Geometry check sheet. Reference: the model listing, model coordinates, mm. A direction names the side the tool comes from. Give positions to 0.01 mm unless a question says otherwise; leave off trailing zeros. Write each loop counter-clockwise with the first axis right and the second up, starting at its lowest first coordinate (ties: lowest second). Pieces come first, ordered by that corner, then holes. Notation, with made-up numbers: (17, -3.5) - (41, -3.5) arc R10 ccw to (41, 14.5) - close; hole circle Ø1 at (30, 48.25). An arc over 180 degrees is marked (long way). One line per question, with ' | ' between items. Start each with the question number.
Q1. Set-up check for faces 1 (the face through (161.076, -36.429, 35.769)), 2 (the face through (66.538, 0.826, -34.608)), 3 (the face through (-129.48, -51.5, 134.64)): record each of +Z, -Z, +X, -X, +Y, -Y from which the full face is reachable in a straight line by a thin tool's end or side.
Q2. Section check B-B on x = -182. Record the boundary of the cut face in (y, z), and give its area (3 significant figures).
Q3. Release check for a two-part mould opening along X. For faces 4 (the face through (-69.12, -51.5, 162.17)), 5 (the face through (-25.532, 11.036, -81.075)), 6 (the face through (-134.64, -51.5, -129.48)), 7 (the face through (118, -56.569, 103)) record: +X half, -X half, draft (parallel to the pull), parting line (faces both ways), or undercut.
Q4. Section check A-A on z = 182. Record the boundary of the cut face in (x, y), and give its area (3 significant figures).
Q5. Section check C-C on y = -32. Record the boundary of the cut face in (x, z), and give its area (3 significant figures).
Q6. Thickness scan on L1, parallel to Y at x = 137.5, z = -113.5; L2, parallel to Y at x = 91, z = 84; L3, parallel to Z at x = 98, y = -16.5. Record the ranges inside material, lowest first. Write a range as [from, to].
Q7. Section check D-D on z = 0. Count the separate pieces of the cut face and the enclosed holes in it, and give its area (3 significant figures).
Q8. Gauge pin test, flat ends, axial feed: P1, Ø8, axis at x = 130, y = -20, coming from the +Z side; P2, Ø10, axis at x = 76.5, z = 120, coming from the +Y side; P3, Ø12, axis at x = 14.5, y = -26, coming from the -Z side. Record the tip position at first contact, or that the pin passes through.
```python
from build123d import *

# Parameters (mm, degrees)
SKETCH3_R          = 6
CUT_EXTRUDE1_DEPTH = 291.215437219
CIRPATTERN1_COUNT  = 16
SKETCH4_R          = 50
CUT_EXTRUDE2_DEPTH = 293.617497768


with BuildPart() as part:
    # Sketch2 → Revolve1 (revolve)
    with BuildSketch(Plane.XY, mode=Mode.PRIVATE) as revolve1_sk:
        with BuildLine():
            Line((155, -56.568542495), (200, -56.568542495))
            Line((200, -56.568542495), (200, -46.568542495))
            Line((200, -46.568542495), (165, -46.568542495))
            Line((165, -46.568542495), (165, -26.568542495))
            ThreePointArc((165, -26.568542495), (156.213203436, -5.355339059), (135, 3.431457505))
            Line((135, 3.431457505), (85, 3.431457505))
            Line((85, 3.431457505), (85, 18.431457505))
            Line((85, 18.431457505), (0, 18.431457505))
            Line((0, 18.431457505), (0, 8.431457505))
            Line((0, 8.431457505), (75, 8.431457505))
            Line((75, 8.431457505), (75, -6.568542495))
            Line((75, -6.568542495), (134.255065141, -6.568542495))
            ThreePointArc((134.255065141, -6.568542495), (148.662982429, -12.382785273), (155, -26.568542495))
            Line((155, -26.568542495), (155, -56.568542495))
        make_face()
    revolve(revolve1_sk.sketch.rotate(Axis((0, 0, 0), (0, 1, 0)), 90), axis=Axis((0, 0, 0), (0, 1, 0)))

    # Sketch3 → Cut-Extrude1 (cut, through all)
    with BuildSketch(Plane(origin=(0, -46.568542495, 0), x_dir=(1, 0, 0), z_dir=(0, 1, 0))):
        with Locations(Location((0, 182, 0), (0, 0, 270))):
            Circle(SKETCH3_R)
    cut_extrude1 = extrude(amount=-CUT_EXTRUDE1_DEPTH, mode=Mode.SUBTRACT)

    # CirPattern1: Cut-Extrude1 ×16 about axis
    cirpattern1_axis = Axis((0, 0, 0), (0, 1, 0))
    for i in range(1, CIRPATTERN1_COUNT):
        add(cut_extrude1.rotate(cirpattern1_axis, i * 360 / CIRPATTERN1_COUNT), mode=Mode.SUBTRACT)

    # Sketch4 → Cut-Extrude2 (cut, through all)
    with BuildSketch(Plane(origin=(0, 18.431457505, 0), x_dir=(1, 0, 0), z_dir=(0, 1, 0))):
        with Locations(Location((0, 0, 0), (0, 0, 270))):
            Circle(SKETCH4_R)
    extrude(amount=-CUT_EXTRUDE2_DEPTH, mode=Mode.SUBTRACT)


solid = part.part
```
Working result:
1) face 1: +Y | face 2: -Y | face 3: +Y, -Y
2) outline: (-56.57, -82.92) - (-46.57, -82.92) - (-46.57, -6) - (-56.57, -6) - close; (-56.57, 6) - (-46.57, 6) - (-46.57, 82.92) - (-56.57, 82.92) - close | area: 1,540 mm2
3) face 4: undercut | face 5: parting line | face 6: undercut | face 7: draft
4) outline: (-82.92, -56.57) - (-6, -56.57) - (-6, -46.57) - (-82.92, -46.57) - close; (6, -56.57) - (82.92, -56.57) - (82.92, -46.57) - (6, -46.57) - close | area: 1,540 mm2
5) outline: circle Ø330 at (0, 0); hole circle Ø310 at (0, 0) | area: 10,100 mm2
6) L1: y = [-56.57, -46.57] | L2: y = [-6.57, 3.43] | L3: z = [-130.57, -116.15], [116.15, 130.57]
7) separate pieces: 4 | enclosed holes: 0 | area: 3,860 mm2
8) P1: stops at z = 105.57 | P2: stops at y = 3.34 | P3: stops at z = -164.78
